Here's how the part is built. I have some questions about the finished solid (model axes, mm). Face numbers are marked on the shaded views. A direction names the side the tool comes from. Coordinates: 2 decimals unless noted, no trailing zeros. Loops run counter-clockwise (first coordinate to the right, second up) from the corner with the lowest first, then second, coordinate; pieces in that order, holes last. Notation, with made-up numbers: (53, -7.5) -> (64, -7.5) arc R20 cw to (64, 6.5) -> close; hole circle Ø10 at (82, 31.5). An arc over 180 degrees is marked (long way). Use CSV: the item, a comma, the result in double quotes. Start each with the question number.
from build123d import *

# Parameters (mm, degrees)
SKETCH1_W           = 19.05
SKETCH1_H           = 50.8
BOSS_EXTRUDE1_DEPTH = 76.2
CUT_EXTRUDE1_REACH  = 78.2
SKETCH2_W           = 12.7
SKETCH2_H           = 44.45
SKETCH4_R           = 8.001
CUT_EXTRUDE2_DEPTH  = 20.05


with BuildPart() as part:
    # Sketch1 → Boss-Extrude1 (new body)
    with BuildSketch(Plane.XY):
        Rectangle(SKETCH1_W, SKETCH1_H)
    extrude(amount=-BOSS_EXTRUDE1_DEPTH)

    # Sketch2 → Cut-Extrude1 (cut, up to next)
    with BuildSketch(Plane.XY, mode=Mode.PRIVATE) as cut_extrude1_sk1:
        Rectangle(SKETCH2_W, SKETCH2_H)
    cut_extrude1_tool1 = extrude(cut_extrude1_sk1.sketch, amount=-CUT_EXTRUDE1_REACH, mode=Mode.PRIVATE) & part.part
    add(cut_extrude1_tool1.solids().sort_by_distance((0, 0, 0))[0], mode=Mode.SUBTRACT)

    # Sketch4 → Cut-Extrude2 (cut, through all)
    with BuildSketch(Plane(origin=(9.525, 0, 0), x_dir=(0, 0, -1), z_dir=(1, 0, 0))):
        with Locations((38.1, -11.049)):
            Circle(SKETCH4_R)
    extrude(amount=-CUT_EXTRUDE2_DEPTH, mode=Mode.SUBTRACT)


solid = part.part
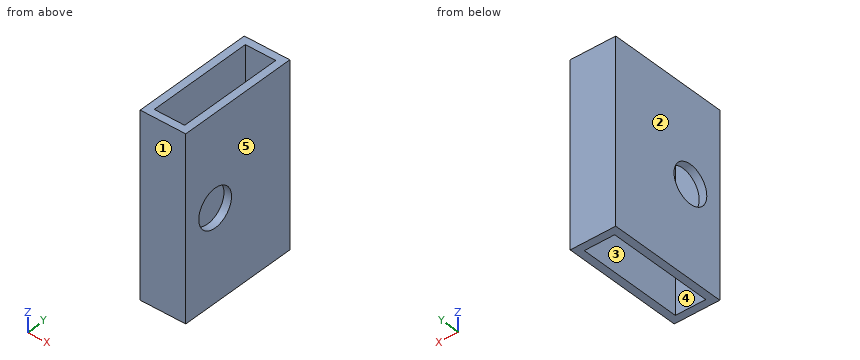
1) Thinking about a two-plate mould opening in X: for the marked faces 1, 2 and 3, which applies, pulls with the +X half, pulls with the -X half, needs draft (parallel to the pull), parting line crosses it, or undercut?
2) Please list where these lines run through material, in increasing order: L1, parallel to X at y = -15.5, z = -53 (3 decimals); L2, parallel to Y at x = 7.1, z = -38.1; L3, parallel to Y at x = 5.5, z = -52 (3 decimals). Write a range as [from, to].
3) I want a section at B-B, the plane z = -38.1. Please give me the cut outline in (x, y) (3 decimals), plus the area to 3 significant figures.
4) Which directions (+Z, -Z, +X, -X, +Y, -Y) give clear straight access to the entire face, cutting with the end or side of a thin tool? Please do the marked faces 4 and 5.
5) I want a section at A-A, the plane x = 5.5. Please give me the cut outline in (y, z) (3 decimals).
6) I want a section at C-C, the plane y = 11.5. Please give me the cut outline in (x, z) (3 decimals), plus the area to 3 significant figures.
7) I want a section at D-D, the plane z = -28. Please give me the cut outline in (x, y) (3 decimals).
Return value:
1,face 1,"needs draft"
1,face 2,"pulls with the -X half"
1,face 3,"undercut"
2,L1,"x = [-9.525, -6.35], [6.35, 9.525]"
2,L2,"y = [-25.4, -19.05], [-3.05, 25.4]"
2,L3,"y = [-25.4, -22.225], [22.225, 25.4]"
3,outline,"(-9.525, -25.4) -> (9.525, -25.4) -> (9.525, -19.05) -> (6.35, -19.05) -> (6.35, -22.225) -> (-6.35, -22.225) -> (-6.35, -19.05) -> (-9.525, -19.05) -> close; (-9.525, -3.048) -> (-6.35, -3.048) -> (-6.35, 22.225) -> (6.35, 22.225) -> (6.35, -3.048) -> (9.525, -3.048) -> (9.525, 25.4) -> (-9.525, 25.4) -> close"
3,area,"302 mm²"
4,face 4,"+Z, -Z"
4,face 5,"+Z, -Z, +X, +Y, -Y"
5,outline,"(-25.4, -76.2) -> (-22.225, -76.2) -> (-22.225, 0) -> (-25.4, 0) -> close; (22.225, -76.2) -> (25.4, -76.2) -> (25.4, 0) -> (22.225, 0) -> close"
6,outline,"(-9.525, -76.2) -> (-6.35, -76.2) -> (-6.35, 0) -> (-9.525, 0) -> close; (6.35, -76.2) -> (9.525, -76.2) -> (9.525, 0) -> (6.35, 0) -> close"
6,area,"484 mm²"
7,outline,"(-9.525, -25.4) -> (9.525, -25.4) -> (9.525, 25.4) -> (-9.525, 25.4) -> close; hole (-6.35, -22.225) -> (6.35, -22.225) -> (6.35, 22.225) -> (-6.35, 22.225) -> close"
